Job drawing, mm, ordinate dimensions from the low corner. One solid piece. Give positions to 0.01 mm unless a question says otherwise; leave off trailing zeros. Write each loop counter-clockwise with the first axis right and the second up, starting at its lowest first coordinate (ties: lowest second). Pieces come first, ordered by that corner, then holes. Notation, with made-up numbers: M 62.5,58 L 118.5,58 A15 ccw 118.5,79 Z; hole C 2.25,-2 d9. An arc over 180 degrees is marked long. Use CSV: the item, a comma, the result in double quotes. Start each with the question number.
Item 1: Cut at C-C (y = 7). List the corners of the cut face in (x, z), then the cut area to 3 significant figures.
Item 2: Drill centre lines: line 1 (X direction, y = 4.75, z = 3); line 2 (X direction, y = 10.5, z = 2.45); line 3 (Z direction, x = 3.6, y = 1.25). Where is each one in solid material? Low to high. Write a range as [from, to].
Item 3: Cut at A-A (x = 3). List the corners of the cut face in (y, z), then the cut area to 3 significant figures.
Item 4: Mould opens along Z. For the marked faces 1, 2 and 3 say: released by +Z, released by -Z, zero draft, split by the parting line, or undercut.
Item 5: Cut at B-B (z = 3). List the corners of the cut face in (x, y), then the cut area to 3 significant figures.
Item 6: Cut at D-D (z = 3.8). List the corners of the cut face in (x, y), then the cut area to 3 significant figures.
Item 7: Pin check, flat tip, straight feed: pin 1 (2.5 mm diameter, centred on x = 3.5, y = 8, fed in from +Z). Stop position of the tip, or through.
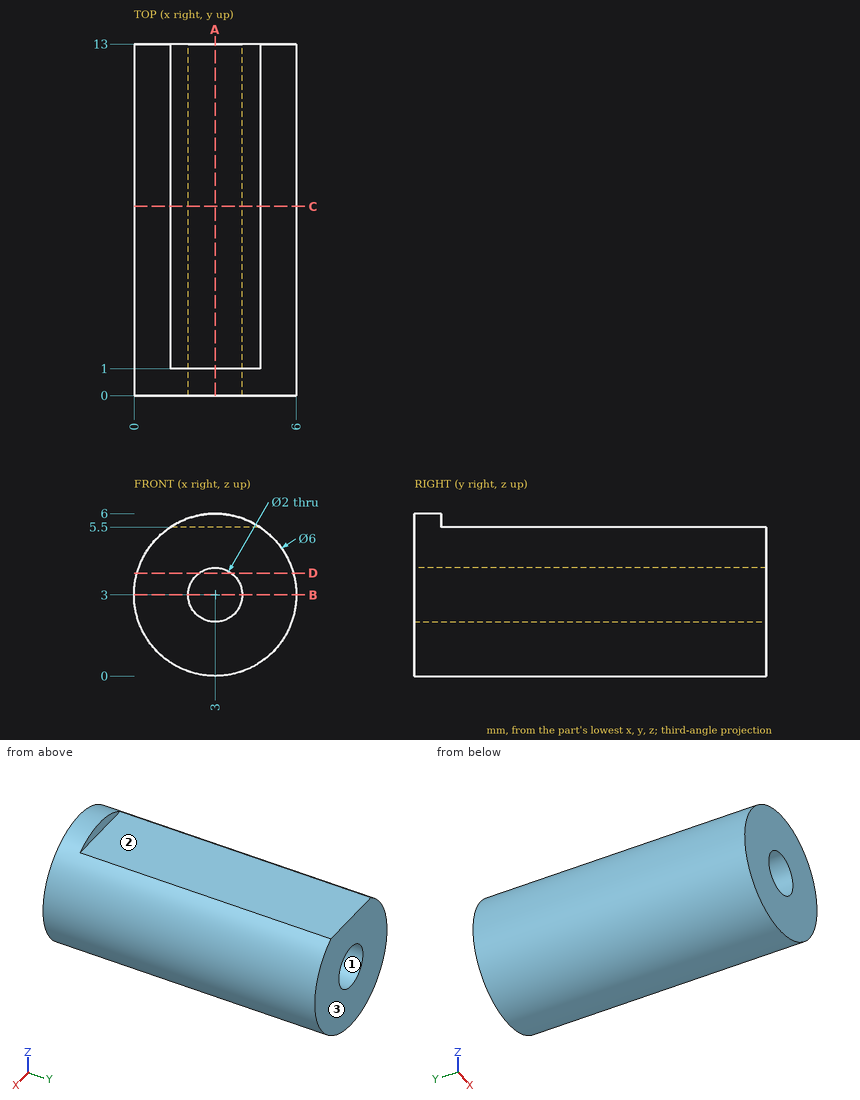
Worked answers:
1,outline,"M 1.34,5.5 A3 ccw long 4.66,5.5 Z; hole C 3,3 d2"
1,area,"24.0 mm^2"
2,line 1,"x = [0, 2], [4, 6]"
2,line 2,"x = [0.05, 2.16], [3.84, 5.95]"
2,line 3,"z = [0.06, 2.2], [3.8, 5.5]"
3,outline,"M 0,0 L 13,0 L 13,2 L 0,2 Z; M 0,4 L 13,4 L 13,5.5 L 1,5.5 L 1,6 L 0,6 Z"
3,area,"46.0 mm^2"
4,face 1,"undercut"
4,face 2,"released by +Z"
4,face 3,"zero draft"
5,outline,"M 0,0 L 2,0 L 2,13 L 0,13 Z; M 4,0 L 6,0 L 6,13 L 4,13 Z"
5,area,"52.0 mm^2"
6,outline,"M 0.11,0 L 2.4,0 L 2.4,13 L 0.11,13 Z; M 3.6,0 L 5.89,0 L 5.89,13 L 3.6,13 Z"
6,area,"59.6 mm^2"
7,pin 1,"stops at z = 5.5"
